from build123d import *

# Parameters (mm, degrees)
SKETCH2_W               = 184
SKETCH2_H               = 332.5
BOSS_EXTRUDE1_DEPTH     = 5
SKETCH3_W               = 36.5
SKETCH3_H               = 5
SKETCH3_W_2             = 62.5
CUT_EXTRUDE1_DEPTH      = 5
CUT_EXTRUDE2_DEPTH      = 10
SKETCH5_R               = 2.1
CUT_EXTRUDE3_DEPTH      = 10
ESQUISSE1_R             = 2.5
ENL_V_MAT_EXTRU_1_DEPTH = 10
ENL_V_MAT_EXTRU_2_DEPTH = 10


with BuildPart() as part:
    # Sketch2 → Boss-Extrude1 (new body)
    with BuildSketch(Plane.XY):
        Rectangle(SKETCH2_W, SKETCH2_H)
    extrude(amount=BOSS_EXTRUDE1_DEPTH)

    # Sketch3 → Cut-Extrude1 (cut)
    with BuildSketch(Plane.XY.offset(5)):
        with Locations((-73.75, -98.75)):
            Rectangle(SKETCH3_W, SKETCH3_H)
        with Locations((60.75, -98.75)):
            Rectangle(SKETCH3_W_2, SKETCH3_H)
        with Locations((-73.75, 163.75)):
            Rectangle(SKETCH3_W, SKETCH3_H)
        with Locations((60.75, 163.75)):
            Rectangle(SKETCH3_W_2, SKETCH3_H)
        with Locations((60.75, 98.75)):
            Rectangle(SKETCH3_W_2, SKETCH3_H)
        with BuildLine():
            Line((27.5, -141.25), (27.5, -166.25))
            Line((27.5, -166.25), (-53.5, -166.25))
            Line((-53.5, -166.25), (-53.5, -141.25))
            ThreePointArc((-53.5, -141.25), (-13, -100.75), (27.5, -141.25))
        make_face()
        with Locations((-73.75, 98.75)):
            Rectangle(SKETCH3_W, SKETCH3_H)
    extrude(amount=-CUT_EXTRUDE1_DEPTH, mode=Mode.SUBTRACT)

    # Sketch4 → Cut-Extrude2 (cut)
    with BuildSketch(Plane.XY.offset(5)):
        Polygon((55.75, 161.25), (55.75, 151.25), (58.65, 151.25), (58.65, 146.25), (62.85, 146.25), (62.85, 151.25), (65.75, 151.25), (65.75, 161.25), align=None)
        Polygon((-78.75, 161.25), (-78.75, 151.25), (-75.85, 151.25), (-75.85, 146.25), (-71.65, 146.25), (-71.65, 151.25), (-68.75, 151.25), (-68.75, 161.25), align=None)
        Polygon((65.75, -166.25), (65.75, -156.25), (62.85, -156.25), (62.85, -151.25), (58.65, -151.25), (58.65, -156.25), (55.75, -156.25), (55.75, -166.25), align=None)
        Polygon((-68.75, -166.25), (-68.75, -156.25), (-71.65, -156.25), (-71.65, -151.25), (-75.85, -151.25), (-75.85, -156.25), (-78.75, -156.25), (-78.75, -166.25), align=None)
    extrude(amount=-CUT_EXTRUDE2_DEPTH, mode=Mode.SUBTRACT)

    # Sketch5 → Cut-Extrude3 (cut)
    with BuildSketch(Plane.XY.offset(5)):
        with Locations((-13, 98.75)):
            Circle(SKETCH5_R)
    extrude(amount=-CUT_EXTRUDE3_DEPTH, mode=Mode.SUBTRACT)

    # Esquisse1 → Enlèv. mat.-Extru.1 (cut)
    with BuildSketch(Plane(origin=(0, 0, 0), x_dir=(-1, 0, 0), z_dir=(0, 0, -1))):
        with Locations((-35.2, -134.33)):
            Circle(ESQUISSE1_R)
        with Locations((-35.2, -124.17)):
            Circle(ESQUISSE1_R)
        with Locations((-84.2, -134.33)):
            Circle(ESQUISSE1_R)
        with Locations((-84.2, -124.17)):
            Circle(ESQUISSE1_R)
        with BuildLine():
            Line((-40.7, -119.25), (-78.7, -119.25))
            ThreePointArc((-78.7, -119.25), (-79.407106781, -119.542893219), (-79.7, -120.25))
            Line((-79.7, -120.25), (-79.7, -138.25))
            ThreePointArc((-79.7, -138.25), (-79.407106781, -138.957106781), (-78.7, -139.25))
            Line((-78.7, -139.25), (-40.7, -139.25))
            ThreePointArc((-40.7, -139.25), (-39.992893219, -138.957106781), (-39.7, -138.25))
            Line((-39.7, -138.25), (-39.7, -120.25))
            ThreePointArc((-39.7, -120.25), (-39.992893219, -119.542893219), (-40.7, -119.25))
        make_face()
    extrude(amount=-ENL_V_MAT_EXTRU_1_DEPTH, mode=Mode.SUBTRACT)

    # Esquisse2 → Enlèv. mat.-Extru.2 (cut)
    with BuildSketch(Plane.XY.offset(5)):
        with BuildLine():
            Line((10.470660362, -8.273773364), (10.470660362, -59.567669296))
            ThreePointArc((10.470660362, -59.567669296), (51.484945295, -58.532619163), (92, -64.995841242))
            Line((92, -64.995841242), (92, -3.75037767))
            ThreePointArc((92, -3.75037767), (50.880784547, 0.378228003), (10.470660362, -8.273773364))
        make_face()
    extrude(amount=-ENL_V_MAT_EXTRU_2_DEPTH, mode=Mode.SUBTRACT)


solid = part.part
Geometry: final body of the model. Coordinates: model frame, mm. A direction names the side the tool comes from. Round coordinates to 2 decimals unless told otherwise and drop trailing zeros. Loops run counter-clockwise (first coordinate to the right, second up) from the corner with the lowest first, then second, coordinate; pieces in that order, holes last.
Q1. Section A-A on y = -146. Return loops of the section in (x, z).
Q2. Section D-D on x = -5. Return loops of the section in (y, z), plus the area to 3 significant figures.
Q3. Section C-C on y = -38.5. Return loops of the section in (x, z).
Q4. Material intervals for L1, parallel to X at y = 152, z = 2.85; L2, parallel to Y at x = -70, z = 0.35; L3, parallel to Y at x = 84.2, z = 2.05, sorted ascending.
Q5. Section B-B on z = 2.95. State how many separate pieces and enclosed holes the cut face has, plus the area to 3 significant figures.
Q6. Pull-direction query (X, two-part tool) for faces 1 (the cylindrical face through (50.911, -58.495, 2.535)), 2 (the flat face through (-1, 2, 0)); classes: released by +X, released by -X, zero draft, split by the parting line, or undercut.
Q7. Access query for faces 3 (the cylindrical face through (51.46, 0.41, 2.54)), 4 (the cylindrical face through (-13.89, -100.76, 2.54)). Directions: +Z, -Z, +X, -X, +Y, -Y. A direction counts if a zero-diameter tool reaches every point of the face in a straight line with its end or side. Return the directions, or none.
Q8. Pin query (flat end, axial travel): P1, Ø2, axis at x = -73.5, z = 2.5, coming from the -Y side; P2, Ø1.5, axis at y = -99.5, z = 2.5, coming from the -X side; P3, Ø2, axis at x = -74.5, z = 1.5, coming from the +Y side. Return the tip coordinate at first contact, or that it passes through.
Evaluation:
1. outline: (-92, 0) - (-53.5, 0) - (-53.5, 5) - (-92, 5) - close; (27.5, 0) - (92, 0) - (92, 5) - (27.5, 5) - close
2. outline: (-101.55, 0) - (166.25, 0) - (166.25, 5) - (-101.55, 5) - close
2. area: 1,340 mm2
3. outline: (-92, 0) - (10.47, 0) - (10.47, 5) - (-92, 5) - close
4. L1: x = -92 to -78.75, -68.75 to 55.75, 65.75 to 92
4. L2: y = -156.25 to -101.25, -96.25 to 96.25, 101.25 to 151.25
4. L3: y = -166.25 to -136.83, -131.83 to -126.67, -121.67 to -101.25, -96.25 to -63.15, -1.96 to 96.25, 101.25 to 161.25
5. separate pieces: 1
5. enclosed holes: 6
5. area: 49,000 mm2
6. face 1: undercut
6. face 2: zero draft
7. face 3: +Z, -Z
7. face 4: +Z, -Z, -Y
8. P1: stops at y = -151.25
8. P2: stops at x = -55.5
8. P3: stops at y = 146.25
